from build123d import *

# Parameters (mm, degrees)
RESSALTO_EXTRUS_O1_DEPTH                             = 500
REBAIXO_PARA_PARAFUSO_DE_CABE_A_SEXTAVAD_D           = 18
REBAIXO_PARA_PARAFUSO_DE_CABE_A_SEXTAVAD_DEPTH       = 58
REBAIXO_PARA_PARAFUSO_DE_CABE_A_SEXTAVAD_CBORE_D     = 26
REBAIXO_PARA_PARAFUSO_DE_CABE_A_SEXTAVAD_CBORE_DEPTH = 25
CHANFRO1_SIZE2                                       = 2.500287455
CHANFRO1_SIZE                                        = 2.500257245
CHANFRO2_SIZE2                                       = 2.500423779
CHANFRO2_SIZE                                        = 2.500287455
CHANFRO3_SIZE                                        = 2


with BuildPart() as part:
    # Esboço1 → Ressalto-extrusão1 (new body)
    with BuildSketch(Plane.XY):
        with BuildLine():
            Line((-31.5, 20.527298986), (-31.5, 0))
            Line((-31.5, 0), (31.5, 0))
            Line((31.5, 0), (31.5, 20.527298986))
            ThreePointArc((31.5, 20.527298986), (28.900076881, 22.150342104), (27.397266061, 24.82156445))
            Line((27.397266061, 24.82156445), (24.5, 25.597882749))
            Line((24.5, 25.597882749), (24.5, 46.397686197))
            Line((24.5, 46.397686197), (27.397119712, 47.17387922))
            ThreePointArc((27.397119712, 47.17387922), (28.898613337, 49.848990738), (31.5, 51.474872705))
            Line((31.5, 51.474872705), (31.5, 58))
            Line((31.5, 58), (-31.5, 58))
            Line((-31.5, 58), (-31.5, 51.474872705))
            ThreePointArc((-31.5, 51.474872705), (-28.899411057, 49.849685923), (-27.397802135, 47.175837466))
            Line((-27.397802135, 47.175837466), (-24.5, 46.399706372))
            Line((-24.5, 46.399706372), (-24.5, 25.596973237))
            Line((-24.5, 25.596973237), (-27.397939574, 24.823365186))
            ThreePointArc((-27.397939574, 24.823365186), (-28.900095464, 22.151244343), (-31.5, 20.527298986))
        make_face()
    extrude(amount=RESSALTO_EXTRUS_O1_DEPTH)

    # Rebaixo para parafuso de cabeça sextavada de M161
    with Locations(Plane(origin=(0, 58, 0), x_dir=(1, 0, 0), z_dir=(0, 1, 0))):
        with Locations((0, -100), (0, -250), (0, -400), (0, -550), (0, -700), (0, -850), (0, -1000), (0, -1150), (0, -1300), (0, -1450), (0, -1600), (0, -1750), (0, -1900), (0, -2050), (0, -2200), (0, -2350)):
            CounterBoreHole(REBAIXO_PARA_PARAFUSO_DE_CABE_A_SEXTAVAD_D / 2, REBAIXO_PARA_PARAFUSO_DE_CABE_A_SEXTAVAD_CBORE_D / 2, REBAIXO_PARA_PARAFUSO_DE_CABE_A_SEXTAVAD_CBORE_DEPTH, depth=REBAIXO_PARA_PARAFUSO_DE_CABE_A_SEXTAVAD_DEPTH)

    # Chanfro1
    chanfro1_edges = [part.edges().sort_by_distance(p)[0] for p in [
        (-31.5, 58, 250),
    ]]
    chamfer(chanfro1_edges, length=CHANFRO1_SIZE, length2=CHANFRO1_SIZE2)

    # Chanfro2
    chanfro2_edges = [part.edges().sort_by_distance(p)[0] for p in [
        (31.5, 58, 250),
    ]]
    chamfer(chanfro2_edges, length=CHANFRO2_SIZE, length2=CHANFRO2_SIZE2)

    # Chanfro3
    chanfro3_edges = [part.edges().sort_by_distance(p)[0] for p in [
        (31.5, 0, 250),
        (-31.5, 0, 250),
    ]]
    chamfer(chanfro3_edges, length=CHANFRO3_SIZE)


solid = part.part
The listing builds one solid part. Answer for the finished solid, in the listing's coordinates (mm). A direction names the side the tool comes from. Give positions to 0.01 mm unless a question says otherwise; leave off trailing zeros. Order: outer loops, then holes, each group sorted by start corner. A loop starts at its lowest first (then second) coordinate and runs counter-clockwise, first axis right, second up. Notation, with made-up numbers: (-22, 55) -> (8, 55) arc R19 ccw to (8, 61) -> close; hole circle Ø4 at (31.5, 11.25). An arc over 180 degrees is marked (long way). Put each result on its own line as item: value.
Item 1: For faces 4 (the face through (3, 33, 391)), 5 (the face through (24.5, 36, 246)), 6 (the face through (-24.5, 36, 246)), determine the directions among +Z, -Z, +X, -X, +Y, -Y from which every point of the face is accessible in a straight line to the end or side of a thin tool.
Established:
face 4: +Y
face 5: +Z, -Z, +X
face 6: +Z, -Z, -X
Item 2: A cutting plane is placed at A-A on z = 100. Give the vertices of the cut face in (x, y), plus the area to 3 significant figures.
Established:
outline: (-31.5, 2) -> (-29.5, 0) -> (-9, 0) -> (-9, 33) -> (-13, 33) -> (-13, 58) -> (-29, 58) -> (-31.5, 55.5) -> (-31.5, 51.47) arc R6.19 cw to (-27.4, 47.18) -> (-24.5, 46.4) -> (-24.5, 25.6) -> (-27.4, 24.82) arc R6.19 cw to (-31.5, 20.53) -> close; (9, 0) -> (29.5, 0) -> (31.5, 2) -> (31.5, 20.53) arc R6.19 cw to (27.4, 24.82) -> (24.5, 25.6) -> (24.5, 46.4) -> (27.4, 47.17) arc R6.19 cw to (31.5, 51.47) -> (31.5, 55.5) -> (29, 58) -> (13, 58) -> (13, 33) -> (9, 33) -> close
area: 2,040 mm^2
Item 3: A cutting plane is placed at B-B on y = 10.5. Give the vertices of the cut face in (x, z).
Established:
outline: (-31.5, 0) -> (31.5, 0) -> (31.5, 500) -> (-31.5, 500) -> close; hole circle Ø18 at (0, 100); hole circle Ø18 at (0, 250); hole circle Ø18 at (0, 400)
Item 4: A cutting plane is placed at C-C on x = -3.5. Give the vertices of the cut face in (y, z).
Established:
outline: (0, 0) -> (58, 0) -> (58, 87.48) -> (33, 87.48) -> (33, 91.71) -> (0, 91.71) -> close; (0, 108.29) -> (33, 108.29) -> (33, 112.52) -> (58, 112.52) -> (58, 237.48) -> (33, 237.48) -> (33, 241.71) -> (0, 241.71) -> close; (0, 258.29) -> (33, 258.29) -> (33, 262.52) -> (58, 262.52) -> (58, 387.48) -> (33, 387.48) -> (33, 391.71) -> (0, 391.71) -> close; (0, 408.29) -> (33, 408.29) -> (33, 412.52) -> (58, 412.52) -> (58, 500) -> (0, 500) -> close
Item 5: For a pull along X with two mould halves and no side action, classify faces 1 (the face through (1.951, 16.269, 108.786)), 2 (the face through (-31.5, 11, 246)), 3 (the face through (13, 58, 246)) as released by +X, released by -X, zero draft, split by the parting line, or undercut.
Established:
face 1: undercut
face 2: released by -X
face 3: zero draft
Item 6: Given P1, Ø5, axis at x = -21, y = 43.5, coming from the -Z side; P2, Ø20.5, axis at x = 0, z = 250, coming from the +Y side; P3, Ø23, axis at y = 32.5, z = 149.5, coming from the -X side; P4, Ø1, axis at y = 49.5, z = 421, coming from the +X side, each flat-ended and moving along its own axis, determine where each tip first touches the part or whether it passes through.
Established:
P1: stops at z = 0
P2: stops at y = 33
P3: stops at x = -30.4
P4: stops at x = 29.05
Item 7: Straight lines are drawn through the part: line 1 (Z direction, x = 0, y = 47); line 2 (Z direction, x = 0, y = 13); line 3 (X direction, y = 22, z = 250). For each, find the intervals that lie inside material, in ascending order.
Established:
line 1: z = 0 to 87, 113 to 237, 263 to 387, 413 to 500
line 2: z = 0 to 91, 109 to 241, 259 to 391, 409 to 500
line 3: x = -29.05 to -9, 9 to 29.05
